from build123d import *

# Parameters (mm, degrees)
F1_DEPTH = 3.5
F2_W     = 0.55
F2_H     = 62.6362580806
F3_DEPTH = 6.1
F4_D     = 3.4


with BuildPart() as f1:
    # F0 (on Right) → F1 (new body)
    with BuildSketch(Plane.YZ):
        Polygon((25.8831996471, 2.85), (-36.7530584335, 2.85), (-36.7530584335, -6.7950769342), (25.8831996471, -6.7950769342), (25.8831996471, 0), align=None)
    extrude(amount=F1_DEPTH)

    # F2 (on face) → F3 (cut)
    with BuildSketch(Plane.XY.offset(2.85)):
        with Locations((1.475, -5.4349293932)):
            Rectangle(F2_W, F2_H)
        with Locations((2.025, -5.4349293932)):
            Rectangle(F2_W, F2_H)
    extrude(amount=-F3_DEPTH, mode=Mode.SUBTRACT)

    # F4 (through all)
    with Locations(Plane(origin=(0, 0, 0), x_dir=(0, 1, 0), z_dir=(-1, 0, 0))):
        with Locations((16.6665, 0), (-33.3333, 0), (0, 0)):
            Hole(F4_D / 2)


solid = f1.part
Check sheet for the modelled part. Datum: model origin and axes. Units: mm. A direction names the side the tool comes from. Give positions to 0.01 mm unless a question says otherwise; leave off trailing zeros. Order: outer loops, then holes, each group sorted by start corner. A loop starts at its lowest first (then second) coordinate and runs counter-clockwise, first axis right, second up. Notation, with made-up numbers: (10, 77.5) - (56, 77.5) arc R30 cw to (56, 109.5) - close; hole circle Ø3 at (12.5, 37). An arc over 180 degrees is marked (long way). Answer as CSV lines item,"result".
1. Section check B-B (y = 0). Record the boundary of the cut face in (x, z).
Result sheet:
outline,"(0, -6.8) - (3.5, -6.8) - (3.5, -1.7) - (2.3, -1.7) - (2.3, -3.25) - (1.2, -3.25) - (1.2, -1.7) - (0, -1.7) - close; (0, 1.7) - (1.2, 1.7) - (1.2, 2.85) - (0, 2.85) - close; (2.3, 1.7) - (3.5, 1.7) - (3.5, 2.85) - (2.3, 2.85) - close"
2. Go/stop test with flat-tipped pins: P1, Ø3, axis at y = 0, z = 0, coming from the -X side; P2, Ø0.5, axis at x = 1.5, y = -8, coming from the +Z side. Record where each tip stops, or that it passes through.
Result sheet:
P1,"through"
P2,"z = -3.25"
3. Section check A-A (z = 0). State how many separate pieces and enclosed holes the cut face has, then the cut area to 3 significant figures.
Result sheet:
separate pieces,"8"
enclosed holes,"0"
area,"126 mm²"
4. Mould release check, pull along Z, two halves, no side actions. Record for faces 1 (the face through (2.3, -6, 0)), 2 (the face through (2.91, 0.37, 1.66)), 3 (the face through (3, -5, 2.85)), 4 (the face through (2.908, 18.365, -0.075)): released by +Z, released by -Z, zero draft, split by the parting line, or undercut.
Result sheet:
face 1,"zero draft"
face 2,"undercut"
face 3,"released by +Z"
face 4,"undercut"
5. Tool access check on faces 5 (the face through (0.608, 18.365, -0.075)), 6 (the face through (2, -5, -3.25)). Record the directions out of +Z, -Z, +X, -X, +Y, -Y that give a thin tool (end or side, any length) a straight path to the whole face; none if there is none.
Result sheet:
face 5,"+X, -X"
face 6,"+Z, +Y, -Y"
6. Section check D-D (y = -10.5). Record the boundary of the cut face in (x, z), then the cut area to 3 significant figures.
Result sheet:
outline,"(0, -6.8) - (3.5, -6.8) - (3.5, 2.85) - (2.3, 2.85) - (2.3, -3.25) - (1.2, -3.25) - (1.2, 2.85) - (0, 2.85) - close"
area,"27.0 mm²"
7. Scan lines: probe 1 along X at (y, z) = (-12, 1); probe 2 along Y at (x, z) = (1.15, -1); probe 3 along Z at (x, y) = (1.6, -12). Record each from-to range of solid material in increasing order. Write a range as from..to.
Result sheet:
probe 1,"0..1.2, 2.3..3.5"
probe 2,"-36.75..-34.71, -31.96..-1.37, 1.37..15.29, 18.04..25.88"
probe 3,"-6.8..-3.25"
8. Section check C-C (x = 0.6). Record the boundary of the cut face in (y, z), then the cut area to 3 significant figures.
Result sheet:
outline,"(-36.75, -6.8) - (25.88, -6.8) - (25.88, 2.85) - (-36.75, 2.85) - close; hole circle Ø3.4 at (-33.33, 0); hole circle Ø3.4 at (0, 0); hole circle Ø3.4 at (16.67, 0)"
area,"577 mm²"
